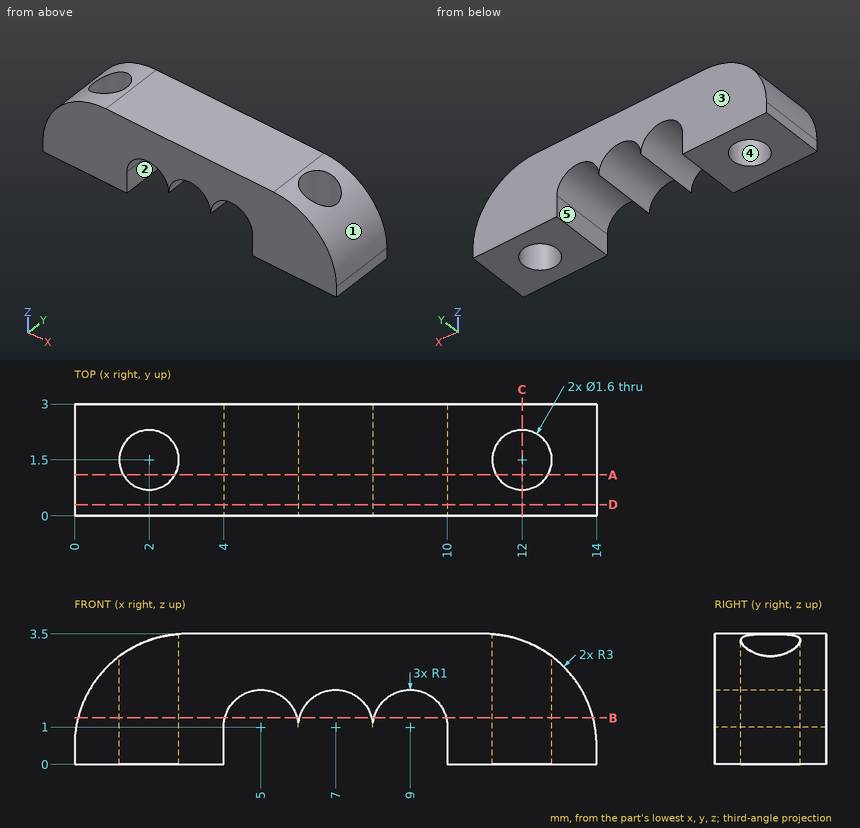
For this review, use the dimensioned drawing (mm, ordinates from the lowest corner) and the shaded views. A direction names the side the tool comes from. Give positions to 0.01 mm unless a question says otherwise; leave off trailing zeros. Write each loop counter-clockwise with the first axis right and the second up, starting at its lowest first coordinate (ties: lowest second). Pieces come first, ordered by that corner, then holes.
(1) Consider section C-C, the plane x = 12. Give the boundary of the cut face in (y, z).
(2) Tool access review of the marked faces 1 and 2: name each direction out of +Z, -Z, +X, -X, +Y, -Y from which nothing blocks a thin tool from reaching the whole face with its end or side.
(3) Consider section D-D, the plane y = 0.3. Give the boundary of the cut face in (x, z), and give its area (3 significant figures).
(4) To check wall thickness, follow L1, parallel to Y at x = 12, z = 1.3; L2, parallel to X at y = 1.95, z = 2.3; L3, parallel to X at y = 1.15, z = 1.6. State the ranges of each line that lie inside material, in increasing order.
(5) The part is to be moulded in two halves that separate along Y. For the marked faces 3, 4 and 5, say which applies: released by +Y, released by -Y, zero draft, split by the parting line, or undercut.
(6) Consider section A-A, the plane y = 1.1. Give the boundary of the cut face in (x, z), and give its area (3 significant figures).
(7) For P1, Ø1.5, axis at x = 8.5, y = 2.5, coming from the -Z side; P2, Ø1.3, axis at x = 12, y = 1.5, coming from the -Z side, all flat-tipped, find the tip position at first contact; note any pin that passes through.
(8) Consider section B-B, the plane z = 1.25. Give the boundary of the cut face in (x, y).
Returned:
1. outline: (0, 0) - (0.7, 0) - (0.7, 3.33) - (0, 3.33) - close; (2.3, 0) - (3, 0) - (3, 3.33) - (2.3, 3.33) - close
2. face 1: +Z, +X, +Y, -Y
2. face 2: -Z, +Y, -Y
3. outline: (0, 0) - (4, 0) - (4, 1) arc R1 cw to (6, 1) arc R1 cw to (8, 1) arc R1 cw to (10, 1) - (10, 0) - (14, 0) - (14, 0.5) arc R3 ccw to (11, 3.5) - (3, 3.5) arc R3 ccw to (0, 0.5) - close
3. area: 34.4 mm2
4. L1: y = 0 to 0.7, 2.3 to 3
4. L2: x = 0.6 to 1.34, 2.66 to 11.34, 12.66 to 13.4
4. L3: x = 0.21 to 1.28, 2.72 to 4.2, 5.8 to 6.2, 7.8 to 8.2, 9.8 to 11.28, 12.72 to 13.79
5. face 3: released by +Y
5. face 4: undercut
5. face 5: zero draft
6. outline: (0, 0) - (1.31, 0) - (1.31, 2.98) arc R3 ccw to (0, 0.5) - close; (2.69, 0) - (4, 0) - (4, 1) arc R1 cw to (6, 1) arc R1 cw to (8, 1) arc R1 cw to (10, 1) - (10, 0) - (11.31, 0) - (11.31, 3.48) arc R3 ccw to (11, 3.5) - (3, 3.5) arc R3 ccw to (2.69, 3.48) - close; (12.69, 0) - (14, 0) - (14, 0.5) arc R3 ccw to (12.69, 2.98) - close
6. area: 25.3 mm2
7. P1: stops at z = 1
7. P2: passes through
8. outline: (0.1, 0) - (4.03, 0) - (4.03, 3) - (0.1, 3) - close; (5.97, 0) - (6.03, 0) - (6.03, 3) - (5.97, 3) - close; (7.97, 0) - (8.03, 0) - (8.03, 3) - (7.97, 3) - close; (9.97, 0) - (13.9, 0) - (13.9, 3) - (9.97, 3) - close; hole circle Ø1.6 at (2, 1.5); hole circle Ø1.6 at (12, 1.5)
